The listing builds one solid part. Answer for the finished solid, in the listing's coordinates (mm). Face numbers are marked on the shaded views. A direction names the side the tool comes from. Give positions to 0.01 mm unless a question says otherwise; leave off trailing zeros. Write each loop counter-clockwise with the first axis right and the second up, starting at its lowest first coordinate (ties: lowest second). Pieces come first, ordered by that corner, then holes. Notation, with made-up numbers: M -11,7.5 L -3,7.5 A17 ccw -3,37.5 Z; hole C -37.75,-16 d6. An arc over 180 degrees is marked long. Return JSON: item names as keys, results as strings.
from build123d import *
from build123d.topology import SkipClean

# Parameters (mm, degrees)
SKETCH1_W               = 40
SKETCH1_H               = 40
SKETCH1_R               = 1.6
SKETCH1_R_2             = 11.25
BOSS_EXTRUDE1_DEPTH     = 8
CHAMFER2_SIZE           = 1
CHAMFER4_SIZE           = 1.3
BOSS_EXTRUDE2_DEPTH     = 5
BOSS_EXTRUDE3_DEPTH     = 40
CUT_EXTRUDE1_DEPTH      = 157.099755039
CUT_EXTRUDE1_DEPTH_BACK = 157.099755039
SKETCH6_W               = 7
SKETCH6_H               = 9.179407211
CUT_EXTRUDE2_START      = -40
SKETCH7_W               = 9.179407211
SKETCH7_H               = 6
CUT_EXTRUDE2_DEPTH      = 40
BOSS_EXTRUDE4_DEPTH     = 10
SKETCH12_W              = 108.011854904
SKETCH12_H              = 137.560499443
CUT_EXTRUDE4_DEPTH      = 165.39530252
SKETCH13_W              = 40
SKETCH13_H              = 6.869500557
BOSS_EXTRUDE7_DEPTH     = 113


with BuildPart() as part:
    # Sketch1 → Boss-Extrude1 (new body)
    with BuildSketch(Plane.XY):
        with Locations((-3.360655738, -3.504098361)):
            Rectangle(SKETCH1_W, SKETCH1_H)
        with Locations((-3.360655738, 12.745901639)):
            Circle(SKETCH1_R, mode=Mode.SUBTRACT)
        with Locations((12.889344262, -3.504098361)):
            Circle(SKETCH1_R, mode=Mode.SUBTRACT)
        with Locations((-3.360655738, -19.754098361)):
            Circle(SKETCH1_R, mode=Mode.SUBTRACT)
        with Locations((-19.610655738, -3.504098361)):
            Circle(SKETCH1_R, mode=Mode.SUBTRACT)
        with Locations((-3.360655738, -3.504098361)):
            Circle(SKETCH1_R_2, mode=Mode.SUBTRACT)
    extrude(amount=BOSS_EXTRUDE1_DEPTH)

    # Chamfer2
    chamfer2_edges = [part.edges().sort_by_distance(p)[0] for p in [
        (-4.960655738, 12.745901639, 0),
        (11.289344262, -3.504098361, 0),
        (-4.960655738, -19.754098361, 0),
        (-21.210655738, -3.504098361, 0),
    ]]
    chamfer(chamfer2_edges, length=CHAMFER2_SIZE)

    # Chamfer4
    chamfer4_edges = [part.edges().sort_by_distance(p)[0] for p in [
        (-14.610655738, -3.504098361, 0),
    ]]
    chamfer(chamfer4_edges, length=CHAMFER4_SIZE)

    # Sketch3 → Boss-Extrude2 (add)
    with SkipClean():  # the faces are left unmerged after this step: merging them gives an invalid solid
        with BuildSketch(Plane.XY.offset(8)):
            with BuildLine():
                Line((-15.860655738, -8.093801966), (-23.360655738, -8.093801966))
                Line((-23.360655738, -8.093801966), (-23.360655738, -23.504098361))
                Line((-23.360655738, -23.504098361), (-7.950359343, -23.504098361))
                Line((-7.950359343, -23.504098361), (-7.950359343, -16.004098361))
                Line((-7.950359343, -16.004098361), (-7.950359343, -13.775277495))
                ThreePointArc((-7.950359343, -13.775277495), (-11.315607026, -11.459049649), (-13.631834872, -8.093801966))
                Line((-13.631834872, -8.093801966), (-15.860655738, -8.093801966))
            make_face()
            with BuildLine():
                Line((-7.950359343, 8.995901639), (-7.950359343, 16.495901639))
                Line((-7.950359343, 16.495901639), (-23.360655738, 16.495901639))
                Line((-23.360655738, 16.495901639), (-23.360655738, 1.085605245))
                Line((-23.360655738, 1.085605245), (-15.860655738, 1.085605245))
                Line((-15.860655738, 1.085605245), (-13.631834872, 1.085605245))
                ThreePointArc((-13.631834872, 1.085605245), (-11.315607026, 4.450852928), (-7.950359343, 6.767080774))
                Line((-7.950359343, 6.767080774), (-7.950359343, 8.995901639))
            make_face()
            with BuildLine():
                Line((16.639344262, 16.495901639), (1.229047868, 16.495901639))
                Line((1.229047868, 16.495901639), (1.229047868, 8.995901639))
                Line((1.229047868, 8.995901639), (1.229047868, 6.767080774))
                ThreePointArc((1.229047868, 6.767080774), (4.594295551, 4.450852928), (6.910523397, 1.085605245))
                Line((6.910523397, 1.085605245), (9.139344262, 1.085605245))
                Line((9.139344262, 1.085605245), (16.639344262, 1.085605245))
                Line((16.639344262, 1.085605245), (16.639344262, 16.495901639))
            make_face()
            with BuildLine():
                Line((16.639344262, -23.504098361), (16.639344262, -8.093801966))
                Line((16.639344262, -8.093801966), (9.139344262, -8.093801966))
                Line((9.139344262, -8.093801966), (6.910523397, -8.093801966))
                ThreePointArc((6.910523397, -8.093801966), (4.594295551, -11.459049649), (1.229047868, -13.775277495))
                Line((1.229047868, -13.775277495), (1.229047868, -16.004098361))
                Line((1.229047868, -16.004098361), (1.229047868, -23.504098361))
                Line((1.229047868, -23.504098361), (16.639344262, -23.504098361))
            make_face()
        extrude(amount=BOSS_EXTRUDE2_DEPTH)

    # Sketch5 → Boss-Extrude3 (add)
    with SkipClean():  # the faces are left unmerged after this step: merging them gives an invalid solid
        with BuildSketch(Plane(origin=(16.639344262, 0, 0), x_dir=(0, 0, -1), z_dir=(1, 0, 0))):
            with BuildLine():
                Line((-13, 16.495901639), (-23, 16.495901639))
                ThreePointArc((-23, 16.495901639), (-30.071067812, 13.566969451), (-33, 6.495901639))
                Line((-33, 6.495901639), (-33, -79.864396018))
                Line((-33, -79.864396018), (-33, -127.934098361))
                Line((-33, -127.934098361), (0, -127.934098361))
                Line((0, -127.934098361), (80, -127.934098361))
                ThreePointArc((80, -127.934098361), (22.298563281, -89.279521012), (0, -23.504098361))
                Line((0, -23.504098361), (-13, -23.504098361))
                Line((-13, -23.504098361), (-13, 16.495901639))
            make_face()
        extrude(amount=-BOSS_EXTRUDE3_DEPTH)

    # Sketch6 → Cut-Extrude1 (cut, two sides: drawn at the far end of the back side and taken through both)
    with SkipClean():  # the faces are left unmerged after this step: merging them gives an invalid solid
        with BuildSketch(Plane(origin=(16.639344262, 0, 0), x_dir=(0, 0, -1), z_dir=(1, 0, 0)).offset(-CUT_EXTRUDE1_DEPTH_BACK)):
            with Locations((-16.5, -3.504098361)):
                Rectangle(SKETCH6_W, SKETCH6_H)
        extrude(amount=CUT_EXTRUDE1_DEPTH + CUT_EXTRUDE1_DEPTH_BACK, mode=Mode.SUBTRACT)

    # Sketch7 → Cut-Extrude2 (cut)
    with SkipClean():  # the faces are left unmerged after this step: merging them gives an invalid solid
        with BuildSketch(Plane(origin=(0, 16.495901639, 0), x_dir=(1, 0, 0), z_dir=(0, 1, 0)).offset(CUT_EXTRUDE2_START)):
            with Locations((-3.360655738, -16)):
                Rectangle(SKETCH7_W, SKETCH7_H)
        extrude(amount=CUT_EXTRUDE2_DEPTH, mode=Mode.SUBTRACT)

    # Sketch8 → Boss-Extrude4 (add)
    with SkipClean():  # the faces are left unmerged after this step: merging them gives an invalid solid
        with BuildSketch(Plane.XZ.offset(127.934098361)):
            Polygon((4.989344262, -32.93820323), (1.139344262, -26.01), (-7.160655738, -26.01), (-11.010655738, -32.93820323), (-7.010655738, -39.866406461), (0.989344262, -39.866406461), align=None)
            Polygon((4.839344262, -52.98679677), (0.839344262, -46.058593539), (-7.160655738, -46.058593539), (-11.160655738, -52.98679677), (-7.160655738, -59.915), (0.839344262, -59.915), align=None)
            Polygon((4.839344262, -13.02898385), (0.839344262, -6.10078062), (-7.160655738, -6.10078062), (-11.160655738, -13.02898385), (-7.160655738, -19.957187081), (0.839344262, -19.957187081), align=None)
            Polygon((4.839344262, 6.97179677), (0.839344262, 13.9), (-7.160655738, 13.9), (-11.160655738, 6.97179677), (-7.160655738, 0.043593539), (0.839344262, 0.043593539), align=None)
        extrude(amount=BOSS_EXTRUDE4_DEPTH)

    # Sketch12 → Cut-Extrude4 (cut, through all)
    with BuildSketch(Plane(origin=(16.639344262, 0, 0), x_dir=(0, 0, -1), z_dir=(1, 0, 0))):
        with Locations((21.005927452, -52.284348083)):
            Rectangle(SKETCH12_W, SKETCH12_H)
    extrude(amount=-CUT_EXTRUDE4_DEPTH, mode=Mode.SUBTRACT)

    # Sketch13 → Boss-Extrude7 (add, through all)
    with BuildSketch(Plane.XY.offset(33)):
        with Locations((-3.360655738, -124.499348083)):
            Rectangle(SKETCH13_W, SKETCH13_H)
    extrude(amount=-BOSS_EXTRUDE7_DEPTH)


solid = part.part
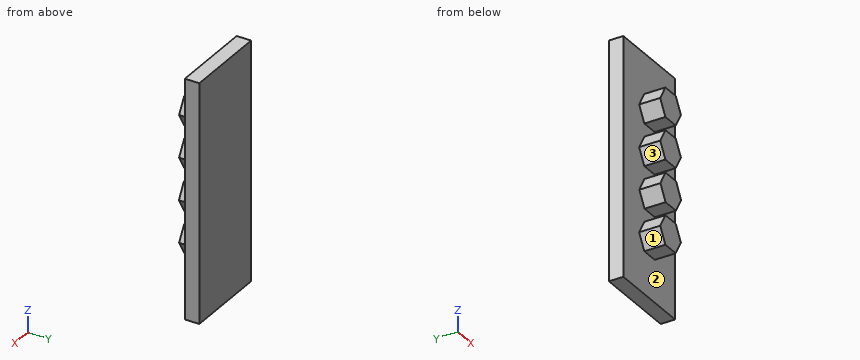
Item 1: A cutting plane is placed at A-A, the plane y = -136.5. Write down the section's boundary in (x, z) (3 decimals), plus the area to 3 significant figures.
Geometry results:
{"outline": "M -11.161,-52.987 L -7.161,-59.915 L 0.839,-59.915 L 4.839,-52.987 L 0.839,-46.059 L -7.161,-46.059 Z; M -11.161,-13.029 L -7.161,-19.957 L 0.839,-19.957 L 4.839,-13.029 L 0.839,-6.101 L -7.161,-6.101 Z; M -11.161,6.972 L -7.161,0.044 L 0.839,0.044 L 4.839,6.972 L 0.839,13.9 L -7.161,13.9 Z; M -11.011,-32.938 L -7.011,-39.866 L 0.989,-39.866 L 4.989,-32.938 L 1.139,-26.01 L -7.161,-26.01 Z", "area": "666 mm2"}
Item 2: A cutting plane is placed at B-B, the plane x = -1.5. Write down the section's boundary in (y, z) (3 decimals).
Geometry results:
{"outline": "M -137.934,-59.915 L -127.934,-59.915 L -127.934,-80 L -121.065,-80 L -121.065,33 L -127.934,33 L -127.934,13.9 L -137.934,13.9 L -137.934,0.044 L -127.934,0.044 L -127.934,-6.101 L -137.934,-6.101 L -137.934,-19.957 L -127.934,-19.957 L -127.934,-26.01 L -137.934,-26.01 L -137.934,-39.866 L -127.934,-39.866 L -127.934,-46.059 L -137.934,-46.059 Z"}
Item 3: Given pin 1 Ø6 at (x, z) = (-13.5, -6) entering from -Y; pin 2 Ø6.5 at (x, y) = (-4, -131.5) entering from +Z; pin 3 Ø2 at (x, y) = (-4.5, -136) entering from -Z (3 decimals); pin 4 Ø5 at (y, z) = (-130, -25.5) entering from +X, each flat-ended and moving along its own axis, determine where each tip first touches the part or whether it passes through.
Geometry results:
{"pin 1": "stops at y = -127.93", "pin 2": "stops at z = 13.9", "pin 3": "stops at z = -59.915", "pin 4": "stops at x = 16.64"}
Item 4: A cutting plane is placed at C-C, the plane z = -64.5. Write down the section's boundary in (x, y).
Geometry results:
{"outline": "M -23.36,-127.93 L 16.64,-127.93 L 16.64,-121.06 L -23.36,-121.06 Z"}
Item 5: Find the intervals of material crossed by line 1 (Z direction, x = 0.5, y = -128.5) (3 decimals); line 2 (Z direction, x = 1, y = -129); line 3 (Y direction, x = -15.5, z = -64.5), in increasing order.
Geometry results:
{"line 1": "z = -59.915 to -46.059, -39.866 to -26.01, -19.957 to -6.101, 0.044 to 13.9", "line 2": "z = -59.64 to -46.34, -39.85 to -26.01, -19.68 to -6.38, 0.32 to 13.62", "line 3": "y = -127.93 to -121.06"}
Item 6: A cutting plane is placed at D-D, the plane x = -17. Write down the section's boundary in (y, z).
Geometry results:
{"outline": "M -127.93,-80 L -121.06,-80 L -121.06,33 L -127.93,33 Z"}
Item 7: Which of the six approach directions +Z, -Z, +X, -X, +Y, -Y give full straight-line access (tool end or side, diameter ignored) to the marked faces 1, 2 and 3?
Geometry results:
{"face 1": "-Z, -X, -Y", "face 2": "-Y", "face 3": "-X, -Y"}
